Input: part model. Units: mm. Frame: model coordinates. A direction names the side the tool comes from. Round coordinates to 2 decimals unless told otherwise and drop trailing zeros. Order: outer loops, then holes, each group sorted by start corner. A loop starts at its lowest first (then second) coordinate and runs counter-clockwise, first axis right, second up. Notation, with made-up numbers: (49, 68.25) -> (71, 68.25) arc R26 ccw to (71, 91.25) -> close; hole circle Ø3 at (44, -31.5). An arc over 180 degrees is marked (long way). Use a Markdown table: item, result.
from build123d import *

# Parameters (mm, degrees)
F1_R     = 7
F1_R_2   = 6
F1_R_3   = 5
F2_DEPTH = 3
F3_DEPTH = 10


# Not quite as in the source:
# - a feature of the source that left no trace in its solid (it failed there, or was rolled back) is left out


with BuildPart() as f2:
    # F1 (on Top) → F2 (new body)
    with BuildSketch(Plane.XY):
        with BuildLine():
            ThreePointArc((9.9107145783, 48.6666821283), (0, 60), (-9.9107145783, 48.6666821283))
            ThreePointArc((-9.9107145783, 48.6666821283), (-25.1057988762, 14.4948397394), (-47.1019403302, -15.7504104697))
            ThreePointArc((-47.1019403302, -15.7504104697), (-51.9615242271, -30), (-37.1912257519, -32.9162716586))
            ThreePointArc((-37.1912257519, -32.9162716586), (0, -28.9896794788), (37.1912257519, -32.9162716586))
            ThreePointArc((37.1912257519, -32.9162716586), (51.9615242271, -30), (47.1019403302, -15.7504104697))
            ThreePointArc((47.1019403302, -15.7504104697), (25.1057988762, 14.4948397394), (9.9107145783, 48.6666821283))
        make_face()
        with Locations((-43.3012701892, -25)):
            Circle(F1_R, mode=Mode.SUBTRACT)
        with Locations((43.3012701892, -25)):
            Circle(F1_R, mode=Mode.SUBTRACT)
        Circle(F1_R_2, mode=Mode.SUBTRACT)
        with Locations((0, 50)):
            Circle(F1_R, mode=Mode.SUBTRACT)
        with Locations((-43.3012701892, -25)):
            Circle(F1_R)
        with Locations((-43.3012701892, -25)):
            Circle(F1_R_3, mode=Mode.SUBTRACT)
        with Locations((43.3012701892, -25)):
            Circle(F1_R)
        with Locations((43.3012701892, -25)):
            Circle(F1_R_3, mode=Mode.SUBTRACT)
        with Locations((0, 50)):
            Circle(F1_R)
        with Locations((0, 50)):
            Circle(F1_R_3, mode=Mode.SUBTRACT)
    extrude(amount=F2_DEPTH)

    # F1 (on Top) → F3 (join)
    with BuildSketch(Plane.XY):
        with BuildLine():
            ThreePointArc((9.9107145783, 48.6666821283), (0, 60), (-9.9107145783, 48.6666821283))
            ThreePointArc((-9.9107145783, 48.6666821283), (-25.1057988762, 14.4948397394), (-47.1019403302, -15.7504104697))
            ThreePointArc((-47.1019403302, -15.7504104697), (-51.9615242271, -30), (-37.1912257519, -32.9162716586))
            ThreePointArc((-37.1912257519, -32.9162716586), (0, -28.9896794788), (37.1912257519, -32.9162716586))
            ThreePointArc((37.1912257519, -32.9162716586), (51.9615242271, -30), (47.1019403302, -15.7504104697))
            ThreePointArc((47.1019403302, -15.7504104697), (25.1057988762, 14.4948397394), (9.9107145783, 48.6666821283))
        make_face()
        with Locations((-43.3012701892, -25)):
            Circle(F1_R, mode=Mode.SUBTRACT)
        with Locations((43.3012701892, -25)):
            Circle(F1_R, mode=Mode.SUBTRACT)
        Circle(F1_R_2, mode=Mode.SUBTRACT)
        with Locations((0, 50)):
            Circle(F1_R, mode=Mode.SUBTRACT)
    extrude(amount=F3_DEPTH)


solid = f2.part
1) Cut plane A-A on y = 50. Return loops of the section in (x, z), and give its area (3 significant figures).
Results found:
| item | result |
|---|---|
| outline | (-10, 0) -> (-5, 0) -> (-5, 3) -> (-7, 3) -> (-7, 10) -> (-10, 10) -> close; (5, 0) -> (10, 0) -> (10, 10) -> (7, 10) -> (7, 3) -> (5, 3) -> close |
| area | 72.0 mm² |
2) Set-up query: faces 1 (the flat face through (-1, -8, 10)), 2 (the flat face through (42, -20, 3)). Return all of +Z, -Z, +X, -X, +Y, -Y with unobstructed straight access to the full face (end or side cutting, diameter ignored); none if empty.
Results found:
| item | result |
|---|---|
| face 1 | +Z, +X, -X, +Y, -Y |
| face 2 | +Z |
3) Cut plane D-D on z = 7.25. Return loops of the section in (x, y).
Results found:
| item | result |
|---|---|
| outline | (-47.1, -15.75) arc R10 ccw (long way) to (-37.19, -32.92) arc R178.09 cw to (37.19, -32.92) arc R10 ccw (long way) to (47.1, -15.75) arc R178.09 cw to (9.91, 48.67) arc R10 ccw (long way) to (-9.91, 48.67) arc R178.09 cw to start; hole circle Ø14 at (-43.3, -25); hole circle Ø14 at (0, 50); hole circle Ø12 at (0, 0); hole circle Ø14 at (43.3, -25) |
4) Line query: L1, parallel to X at y = -25, z = 5; L2, parallel to X at y = -23.5, z = 4.5; L3, parallel to Y at x = -4.5, z = 6.5. Output: solid intervals per line, ascending. Write a range as [from, to].
Results found:
| item | result |
|---|---|
| L1 | x = [-53.3, -50.3], [-36.3, 36.3], [50.3, 53.3] |
| L2 | x = [-53.19, -50.14], [-36.46, 36.46], [50.14, 53.19] |
| L3 | y = [-29.05, -3.97], [3.97, 44.64], [55.36, 58.93] |
5) Cut plane C-C on y = -25. Return loops of the section in (x, z), and give its area (3 significant figures).
Results found:
| item | result |
|---|---|
| outline | (-53.3, 0) -> (-48.3, 0) -> (-48.3, 3) -> (-50.3, 3) -> (-50.3, 10) -> (-53.3, 10) -> close; (-38.3, 0) -> (38.3, 0) -> (38.3, 3) -> (36.3, 3) -> (36.3, 10) -> (-36.3, 10) -> (-36.3, 3) -> (-38.3, 3) -> close; (48.3, 0) -> (53.3, 0) -> (53.3, 10) -> (50.3, 10) -> (50.3, 3) -> (48.3, 3) -> close |
| area | 810 mm² |
6) Cut plane B-B on x = 0. Return loops of the section in (y, z).
Results found:
| item | result |
|---|---|
| outline | (-28.99, 0) -> (-6, 0) -> (-6, 10) -> (-28.99, 10) -> close; (6, 0) -> (45, 0) -> (45, 3) -> (43, 3) -> (43, 10) -> (6, 10) -> close; (55, 0) -> (60, 0) -> (60, 10) -> (57, 10) -> (57, 3) -> (55, 3) -> close |
7) Pin query (flat end, axial travel): pin 1 Ø3 at (x, z) = (24, 2) entering from -Y; pin 2 Ø5 at (x, z) = (-32.5, 2) entering from -Y. Return the tip coordinate at first contact, or that it passes through.
Results found:
| item | result |
|---|---|
| pin 1 | stops at y = -30.82 |
| pin 2 | stops at y = -32.46 |
8) Pull-direction query (Y, two-part tool) for faces 3 (the cylindrical face through (-0.52, -28.99, 4.93)), 4 (the cylindrical face through (-38.683, -26.915, 1.479)), 5 (the flat face through (-45, -20, 3)), 6 (the flat face through (-1, -8, 0)); classes: +Y half, -Y half, draft (parallel to the pull), parting line (faces both ways), or undercut.
Results found:
| item | result |
|---|---|
| face 3 | -Y half |
| face 4 | undercut |
| face 5 | undercut |
| face 6 | draft |
